Part model, mm, in its own coordinate system. Face numbers are marked on the shaded views. A direction names the side the tool comes from. Coordinates: 2 decimals unless noted, no trailing zeros. Order: outer loops, then holes, each group sorted by start corner. A loop starts at its lowest first (then second) coordinate and runs counter-clockwise, first axis right, second up. Notation, with made-up numbers: (59, -9.75) - (95, -9.75) arc R19 ccw to (95, 12.25) - close; hole circle Ø3 at (78.25, 6.25). An arc over 180 degrees is marked (long way). Use a Markdown table: item, result. Add a question column.
1) Saw through at A-A on z = -1.5. List the corners of the cut face in (x, y).
2) Saw through at D-D on z = -3.25. List the corners of the cut face in (x, y), then the cut area to 3 significant figures.
3) Wall check: L1, parallel to Y at x = 6, z = -0.5; L2, parallel to X at y = 1.25, z = -0.5; L3, parallel to Y at x = -5.5, z = -2.5. Give the ranges that are in metal, low to high. Write a range as [from, to].
4) Saw through at C-C on y = 7.25. List the corners of the cut face in (x, z).
5) Two-plate mould, pull along X, no slides. Class the marked faces 1, 2 and 3: +X half, -X half, draft (parallel to the pull), parting line (faces both ways), or undercut.
6) Drop a flat-ended pin along its axis: P1, Ø1.3, axis at x = 6, y = 7.25, coming from the -Z side. Give the stop position or say it passes through.
7) Tool access for the marked faces 4 and 5: list every direction of +Z, -Z, +X, -X, +Y, -Y with a clear straight run to the whole face (end or side of a thin tool).
8) Saw through at B-B on x = -6. List the corners of the cut face in (y, z).
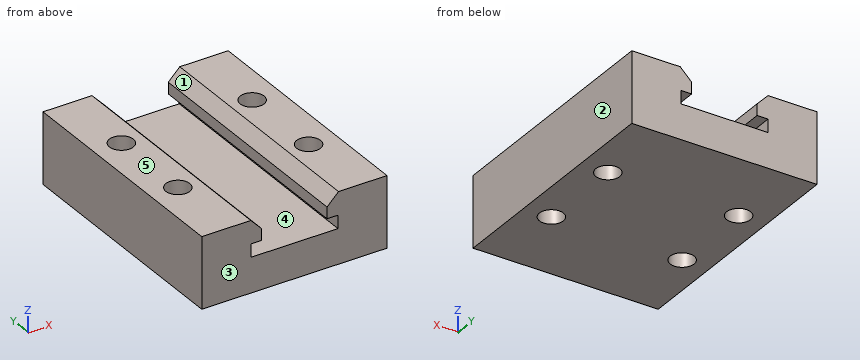
```python
from build123d import *

# Parameters (mm, degrees)
EXTRUDE_1_DEPTH     = 22.5
SKETCH_2_R          = 1.1
CUT_EXTRUDE_1_DEPTH = 10


with BuildPart() as part:
    # 草图1 → 凸台-拉伸1 (new body)
    with BuildSketch(Plane(origin=(0, 0, 0), x_dir=(1, 0, 0), z_dir=(0, 1, 0))):
        Polygon((-4, 0.824883125), (-3, 0.824883125), (-3, -0.225116875), (-4, -1.275116875), (-8.5, -1.275116875), (-8.5, 5.224883125), (8.5, 5.224883125), (8.5, -1.275116875), (4.05, -1.275116875), (3, -0.225116875), (3, 0.824883125), (4, 0.824883125), (4, 2.024883125), (-4, 2.024883125), align=None)
    extrude(amount=EXTRUDE_1_DEPTH)

    # 草图2 → 切除-拉伸1 (cut)
    with BuildSketch(Plane(origin=(0, 0, -5.224883125), x_dir=(-1, 0, 0), z_dir=(0, 0, -1))):
        with Locations((-6, 15.25)):
            Circle(SKETCH_2_R)
        with Locations((6, 15.25)):
            Circle(SKETCH_2_R)
        with Locations((6, 7.25)):
            Circle(SKETCH_2_R)
        with Locations((-6, 7.25)):
            Circle(SKETCH_2_R)
    extrude(amount=-CUT_EXTRUDE_1_DEPTH, mode=Mode.SUBTRACT)


solid = part.part
```
Results are:
| question | item | result |
|---|---|---|
| 1 | outline | (-8.5, 0) - (-4, 0) - (-4, 22.5) - (-8.5, 22.5) - close; (4, 0) - (8.5, 0) - (8.5, 22.5) - (4, 22.5) - close; hole circle Ø2.2 at (-6, 7.25); hole circle Ø2.2 at (-6, 15.25); hole circle Ø2.2 at (6, 7.25); hole circle Ø2.2 at (6, 15.25) |
| 2 | outline | (-8.5, 0) - (8.5, 0) - (8.5, 22.5) - (-8.5, 22.5) - close; hole circle Ø2.2 at (-6, 7.25); hole circle Ø2.2 at (-6, 15.25); hole circle Ø2.2 at (6, 7.25); hole circle Ø2.2 at (6, 15.25) |
| 2 | area | 367 mm2 |
| 3 | L1 | [0, 6.15], [8.35, 14.15], [16.35, 22.5] |
| 3 | L2 | [-8.5, -3], [3, 8.5] |
| 3 | L3 | [0, 6.27], [8.23, 14.27], [16.23, 22.5] |
| 4 | outline | (-8.5, -5.22) - (-7.1, -5.22) - (-7.1, 1.28) - (-8.5, 1.28) - close; (-4.9, -5.22) - (4.9, -5.22) - (4.9, 1.28) - (4.05, 1.28) - (3, 0.23) - (3, -0.82) - (4, -0.82) - (4, -2.02) - (-4, -2.02) - (-4, -0.82) - (-3, -0.82) - (-3, 0.23) - (-4, 1.28) - (-4.9, 1.28) - close; (7.1, -5.22) - (8.5, -5.22) - (8.5, 1.28) - (7.1, 1.28) - close |
| 5 | face 1 | undercut |
| 5 | face 2 | +X half |
| 5 | face 3 | draft |
| 6 | P1 | through |
| 7 | face 4 | +Y, -Y |
| 7 | face 5 | +Z, +X, -X, +Y, -Y |
| 8 | outline | (0, -5.22) - (6.15, -5.22) - (6.15, 1.28) - (0, 1.28) - close; (8.35, -5.22) - (14.15, -5.22) - (14.15, 1.28) - (8.35, 1.28) - close; (16.35, -5.22) - (22.5, -5.22) - (22.5, 1.28) - (16.35, 1.28) - close |
